Source: CAD feature listing. Evaluate the final solid. Frame: model axes, mm. A direction names the side the tool comes from. Give positions to 0.01 mm unless a question says otherwise; leave off trailing zeros. Order: outer loops, then holes, each group sorted by start corner. A loop starts at its lowest first (then second) coordinate and runs counter-clockwise, first axis right, second up. Notation, with made-up numbers: (80.5, 41.5) - (127.5, 41.5) arc R7 ccw to (127.5, 51.5) - close; hole circle Ø10 at (63.5, 44). An arc over 180 degrees is marked (long way). Write each question's results on one line, items separated by ' | '. Start each with the question number.
Item 1: Section A-A on y = -0.8. Output: boundary loops of the cut face in (x, z), and give its area (3 significant figures).
Item 2: Mould query, pull axis X, two halves, no side actions, for faces 1 (the flat face through (16.3, 0, -48)), 2 (the flat face through (3, 1.25, 3)), 3 (the flat face through (0, 1, -97.5)). Classes: released by +X, released by -X, zero draft, split by the parting line, or undercut.
Item 3: Contact query for flat-ended pins moving along their axis: pin 1 Ø13 at (x, z) = (-5.5, -52) entering from -Y; pin 2 Ø3.5 at (x, z) = (0, 0.5) entering from -Y; pin 3 Ø0.5 at (x, y) = (-1, 1.5) entering from +Z; pin 4 Ø5 at (x, z) = (-12.5, -45.5) entering from -Y. Output: stop coordinate, or through.
Item 4: Section D-D on x = -10. Output: boundary loops of the cut face in (y, z), and give its area (3 significant figures).
Item 5: Section B-B on x = 0. Output: boundary loops of the cut face in (y, z), and give its area (3 significant figures).
Item 6: Set-up query: faces 4 (the flat face through (-1, 1, -62)), 5 (the flat face through (-15, -2.5, -37)), 6 (the flat face through (0, -1.5, 0)). Return all of +Z, -Z, +X, -X, +Y, -Y with unobstructed straight access to the full face (end or side cutting, diameter ignored); none if empty.
Item 7: Section C-C on z = -88.5. Output: boundary loops of the cut face in (x, y).
Item 8: Line query: line 1 along X through (y, z) = (0.95, 0); line 2 along Z through (x, y) = (0, 0.75); line 3 along Z through (x, y) = (7.5, 0.35). Output: solid intervals per line, ascending.
Autodesk Fusion 360 part; units mm, degrees
sketch "Sketch1" plane through (0, 0, 0) normal (0, 1, 0) x (1, 0, 0)
  line L0 (-16.3, 0) -> (16.3, 0)
  line L1 (16.3, 0) -> (16.3, 97.5)
  line L2 (16.3, 97.5) -> (-16.3, 97.5)
  line L3 (-16.3, 97.5) -> (-16.3, 0)
  line L4 (0, 102.6744) -> (0, -20) construction
  arc A0 (-16.3, 0) -> (16.3, 0) centre (0, 0) ccw
  line L5 (-14.35, 97.5) -> (-14.35, 0)
  arc A1 (-14.35, 0) -> (14.35, 0) centre (0, 0) ccw
  line L6 (14.35, 0) -> (14.35, 97.5)
  dimension "d1" = 32.6
  dimension "d2" = 97.5
  dimension "d3" = 1.95
extrude "Extrude1" add sketch "Sketch1" along normal blind 2
extrude "Extrude2" add sketch "Sketch1" against normal blind 2.5 contours L0 L2 L3 L5 | L0 A0 A1 | L0 L1 L2 L6
sketch "Sketch2" plane through (0, 0, 7.15) normal (0, 1, 0) x (1, 0, 0)
  circle A0 centre (0, 7.15) radius 3.5
  circle A1 centre (0, 7.15) radius 4.1
  circle A2 centre (0, 7.15) radius 4.7
  circle A3 centre (0, 7.15) radius 5.3
  circle A4 centre (0, 7.15) radius 5.9
  circle A5 centre (0, 7.15) radius 6.5
  circle A6 centre (0, 7.15) radius 7.1
  circle A7 centre (0, 7.15) radius 7.7
  circle A8 centre (0, 7.15) radius 8.3
  line L0 (27.1083, -9.4638) -> (28.3083, -9.4638)
  line L1 (28.3083, -9.4638) -> (28.3083, -7.488)
  line L2 (28.3083, -7.488) -> (27.1083, -7.488)
  line L3 (27.1083, -7.488) -> (27.1083, -9.4638)
  circle A9 centre (0, 7.15) radius 8.9
  circle A10 centre (0, 7.15) radius 9.5
  circle A11 centre (0, 7.15) radius 10.1
  circle A12 centre (0, 7.15) radius 10.7
  circle A13 centre (0, 7.15) radius 11.3
  circle A14 centre (0, 7.15) radius 11.9
  circle A15 centre (0, 7.15) radius 12.5
  dimension "d18" = 7
  dimension "d19" = 8.2
  dimension "d20" = 1.2
  dimension "d21" = 9.4
  dimension "d22" = 10.6
  dimension "d23" = 11.8
  dimension "d24" = 13
  dimension "d25" = 14.2
  dimension "d26" = 15.4
  dimension "d27" = 16.6
  dimension "d28" = 17.8
  dimension "d29" = 19
  dimension "d30" = 20.2
  dimension "d31" = 21.4
  dimension "d32" = 22.6
  dimension "d33" = 23.8
  dimension "d34" = 25
extrude "Extrude4" cut sketch "Sketch2" along normal blind 1.25 contours A1 | A2 | A3 | A4 | A5 | A6 | A7 | A8 | A9 | A10 | A11 | A12 | A13 | A14 | A15
extrude "Extrude5" add 1 faces at (0.555, 0, 0.9381) along direction (0, -1, 0) blind 1.5
sketch "Sketch3" plane through (0, 0, 0) normal (0, -1, 0) x (1, 0, 0)
  line L0 (14.35, -97.5) -> (14.35, 0)
  arc A0 (14.35, 0) -> (-14.35, 0) centre (0, 0) ccw
  line L1 (-14.35, 0) -> (-14.35, -97.5)
  line L2 (-14.35, -97.5) -> (14.35, -97.5)
  circle A1 centre (0, 0) radius 12.5
  line L3 (13, -62.5) -> (-13, -62.5)
  line L4 (-13, -62.5) -> (-13, -46.5)
  line L5 (-13, -46.5) -> (13, -46.5)
  line L6 (13, -46.5) -> (13, -62.5)
  line L7 (13, -62.5) -> (-13, -46.5) construction
  line L8 (-13, -62.5) -> (13, -46.5) construction
  dimension "d39" = 26
  dimension "d40" = 16
  dimension "d41" = 35
extrude "Extrude6" cut sketch "Sketch3" against normal blind 1 contours L3 L4 L5 L6
sketch "Sketch4" plane through (0, 1, 0) normal (0, -1, 0) x (1, 0, 0)
  line L0 (13, -46.5) -> (-13, -46.5)
  line L1 (-13, -46.5) -> (-13, -62.5)
  line L2 (-13, -62.5) -> (13, -62.5)
  line L3 (13, -62.5) -> (13, -46.5)
  line L4 (11.8, -61.3) -> (-11.8, -61.3)
  line L5 (-11.8, -61.3) -> (-11.8, -47.7)
  line L6 (-11.8, -47.7) -> (11.8, -47.7)
  line L7 (11.8, -47.7) -> (11.8, -61.3)
  line L8 (11.8, -61.3) -> (-11.8, -47.7) construction
  line L9 (-11.8, -61.3) -> (11.8, -47.7) construction
  dimension "d44" = 23.6
  dimension "d45" = 13.6
extrude "Extrude7" cut sketch "Sketch4" against normal blind 1 contours L4 L5 L6 L7
equation "d1 = 33 mm - 0.4 mm"
equation "d2 = 114 mm - ( 33 / 2 ) * 1 mm"
equation "d19 = d18 + d20"
equation "d21 = d19 + d20"
equation "d22 = d21 + d20"
equation "d23 = d22 + d20"
equation "d24 = d23 + d20"
equation "d25 = d24 + d20"
equation "d26 = d25 + d20"
equation "d27 = d26 + d20"
equation "d28 = d27 + d20"
equation "d29 = d28 + d20"
equation "d30 = d29 + d20"
equation "d31 = d30 + d20"
equation "d32 = d31 + d20"
equation "d33 = d32 + d20"
equation "d34 = d33 + d20"
Evaluation:
1) outline: (-16.3, -97.5) - (-14.35, -97.5) - (-14.35, 0) arc R14.35 cw to (14.35, 0) - (14.35, -97.5) - (16.3, -97.5) - (16.3, 0) arc R16.3 ccw to (-16.3, 0) - close; circle Ø7 at (0, 0) | area: 513 mm^2
2) face 1: released by +X | face 2: undercut | face 3: zero draft
3) pin 1: stops at y = 0 | pin 2: stops at y = -1.5 | pin 3: stops at z = 16.28 | pin 4: stops at y = -2.5
4) outline: (-2.5, 10.29) - (0, 10.29) - (0, 7.5) - (1.25, 7.5) - (1.25, -7.5) - (0, -7.5) - (0, -46.5) - (1, -46.5) - (1, -47.7) - (2, -47.7) - (2, 12.87) - (-2.5, 12.87) - close; (0, -97.5) - (2, -97.5) - (2, -61.3) - (1, -61.3) - (1, -62.5) - (0, -62.5) - close | area: 179 mm^2
5) outline: (-2.5, 14.35) - (0, 14.35) - (0, 12.5) - (1.25, 12.5) - (1.25, 3.5) - (-1.5, 3.5) - (-1.5, -3.5) - (1.25, -3.5) - (1.25, -12.5) - (0, -12.5) - (0, -46.5) - (1, -46.5) - (1, -47.7) - (2, -47.7) - (2, 16.3) - (-2.5, 16.3) - close; (0, -97.5) - (2, -97.5) - (2, -61.3) - (1, -61.3) - (1, -62.5) - (0, -62.5) - close | area: 191 mm^2
6) face 4: -Y | face 5: +Z, -Z, +X, -X, -Y | face 6: -Z, -Y
7) outline: (-16.3, -2.5) - (-14.35, -2.5) - (-14.35, 0) - (14.35, 0) - (14.35, -2.5) - (16.3, -2.5) - (16.3, 2) - (-16.3, 2) - close
8) line 1: x = -16.3 to -12.5, -3.5 to 3.5, 12.5 to 16.3 | line 2: z = -97.5 to -62.5, -46.5 to -12.5, -3.5 to 3.5, 12.5 to 16.3 | line 3: z = -97.5 to -62.5, -46.5 to -10, 10 to 14.47
